```python
from build123d import *

# Parameters (mm, degrees)
PAD002_DEPTH              = 7.5
BODY002_PLACEMENT_ANGLE   = 90
CYLINDER015_R             = 4.5
CYLINDER015_DEPTH         = 9.5
COMPOUND_PLACEMENT_ANGLE  = 30
CYLINDER014_R             = 4.5
CYLINDER014_DEPTH         = 9.5
PAD001_DEPTH              = 4
BODY001_PLACEMENT_ANGLE   = 90
PAD_DEPTH                 = 7.5
BODY_PLACEMENT_ANGLE      = 90
CYLINDER016_R             = 2.25
CYLINDER016_DEPTH         = 9.5
BOX002_W                  = 58.914519
BOX002_H                  = 9.5
BOX002_DEPTH              = 15
BOX_W                     = 22
BOX_H                     = 9.5
BOX_DEPTH                 = 80.829038
CYLINDER013_R             = 11
CYLINDER013_DEPTH         = 9.5
CYLINDER012_R             = 11
CYLINDER012_DEPTH         = 9.5
FUSION005_PLACEMENT_ANGLE = 30
BOX001_W                  = 22
BOX001_H                  = 9.5
BOX001_DEPTH              = 50
FILLET_R                  = 2
FILLET001_R               = 2
FILLET002_R               = 2


with BuildPart() as m8press001:
    # Sketch002 → Pad002 (new body)
    with BuildSketch(Plane.XY):
        Polygon((7.5, 0), (3.75, 6.495191), (-3.75, 6.495191), (-7.5, 0), (-3.75, -6.495191), (3.75, -6.495191), align=None)
    extrude(amount=PAD002_DEPTH)


with BuildPart() as m8press001_1:
    # Body002 placement: moved
    add(m8press001.part.moved(Location((40.414519, -2, 70))).rotate(Axis((40.414519, -2, 70), (1, 0, 0)), BODY002_PLACEMENT_ANGLE))


with BuildPart() as compound:
    # Cylinder015 → Cylinder015 (new body)
    with BuildSketch(Plane(origin=(0, 0, 81), x_dir=(1, 0, 0), z_dir=(0, -1, 0))):
        Circle(CYLINDER015_R)
    extrude(amount=CYLINDER015_DEPTH)


with BuildPart() as compound_1:
    # Compound placement: moved
    add(compound.part.rotate(Axis((0, 0, 0), (0, 1, 0)), COMPOUND_PLACEMENT_ANGLE))


with BuildPart() as cylinder014:
    # Cylinder014 → Cylinder014 (new body)
    with BuildSketch(Plane.XZ):
        Circle(CYLINDER014_R)
    extrude(amount=CYLINDER014_DEPTH)


with BuildPart() as m4press:
    # Sketch001 → Pad001 (new body)
    with BuildSketch(Plane.XY):
        Polygon((4, 0), (2, 3.464102), (-2, 3.464102), (-4, 0), (-2, -3.464102), (2, -3.464102), align=None)
    extrude(amount=PAD001_DEPTH)


with BuildPart() as m4press_1:
    # Body001 placement: moved
    add(m4press.part.moved(Location((0, -5.5, 112.5))).rotate(Axis((0, -5.5, 112.5), (1, 0, 0)), BODY001_PLACEMENT_ANGLE))


with BuildPart() as m8press:
    # Sketch → Pad (new body)
    with BuildSketch(Plane.XY):
        Polygon((7.5, 0), (3.75, 6.495191), (-3.75, 6.495191), (-7.5, 0), (-3.75, -6.495191), (3.75, -6.495191), align=None)
    extrude(amount=PAD_DEPTH)


with BuildPart() as m8press_1:
    # Body placement: moved
    add(m8press.part.rotate(Axis((0, 0, 0), (1, 0, 0)), BODY_PLACEMENT_ANGLE))


with BuildPart() as fusion006:
    # Cylinder016 → Cylinder016 (new body)
    with BuildSketch(Plane(origin=(0, 0, 112.5), x_dir=(1, 0, 0), z_dir=(0, -1, 0))):
        Circle(CYLINDER016_R)
    extrude(amount=CYLINDER016_DEPTH)

    # Fusion006: union M8Press001, Compound, Cylinder014, M4Press, M8Press
    add(m8press001_1.part)
    add(compound_1.part)
    add(cylinder014.part)
    add(m4press_1.part)
    add(m8press_1.part)


with BuildPart() as cube002:
    # Box002 → Box002 (new body)
    with BuildSketch(Plane(origin=(-7.5, -9.5, 105), x_dir=(1, 0, 0), z_dir=(0, 0, 1))):
        with Locations((29.457259, 4.75)):
            Rectangle(BOX002_W, BOX002_H)
    extrude(amount=BOX002_DEPTH)


with BuildPart() as cube:
    # Box → Box (new body)
    with BuildSketch(Plane(origin=(-11, -9.5, 0), x_dir=(1, 0, 0), z_dir=(0, 0, 1))):
        with Locations((11, 4.75)):
            Rectangle(BOX_W, BOX_H)
    extrude(amount=BOX_DEPTH)


with BuildPart() as cylinder013:
    # Cylinder013 → Cylinder013 (new body)
    with BuildSketch(Plane(origin=(0, 0, 81), x_dir=(1, 0, 0), z_dir=(0, -1, 0))):
        Circle(CYLINDER013_R)
    extrude(amount=CYLINDER013_DEPTH)


with BuildPart() as fusion005:
    # Cylinder012 → Cylinder012 (new body)
    with BuildSketch(Plane.XZ):
        Circle(CYLINDER012_R)
    extrude(amount=CYLINDER012_DEPTH)

    # Fusion005: union Cube, Cylinder013
    add(cube.part)
    add(cylinder013.part)


with BuildPart() as fusion005_1:
    # Fusion005 placement: moved
    add(fusion005.part.rotate(Axis((0, 0, 0), (0, 1, 0)), FUSION005_PLACEMENT_ANGLE))


with BuildPart() as fillet002:
    # Box001 → Box001 (new body)
    with BuildSketch(Plane(origin=(29.414519, -9.5, 70), x_dir=(1, 0, 0), z_dir=(0, 0, 1))):
        with Locations((11, 4.75)):
            Rectangle(BOX001_W, BOX001_H)
    extrude(amount=BOX001_DEPTH)

    # Fusion007: union Cube002, Fusion005
    add(cube002.part)
    add(fusion005_1.part)

    # Cut005: cut Fusion006
    add(fusion006.part, mode=Mode.SUBTRACT)

    # Fillet
    fillet_edges = [fillet002.edges().sort_by_distance(p)[0] for p in [
        (51.414519, -4.75, 120),
        (-7.5, -4.75, 105),
        (-7.5, -4.75, 120),
    ]]
    fillet(fillet_edges, radius=FILLET_R)

    # Fillet001
    fillet001_edges = [fillet002.edges().sort_by_distance(p)[0] for p in [
        (29.414519, -4.75, 105),
    ]]
    fillet(fillet001_edges, radius=FILLET001_R)

    # Fillet002
    fillet002_edges = [fillet002.edges().sort_by_distance(p)[0] for p in [
        (29.414519, -4.75, 72.947441),
    ]]
    fillet(fillet002_edges, radius=FILLET002_R)


solid = fillet002.part
```
Build history of the part. All positions in model axes, mm. A direction names the side the tool comes from. Coordinates: 2 decimals unless noted, no trailing zeros. Order: outer loops, then holes, each group sorted by start corner. A loop starts at its lowest first (then second) coordinate and runs counter-clockwise, first axis right, second up. Notation, with made-up numbers: (30.5, -6) -> (44.5, -6) arc R35 ccw to (44.5, 28) -> close; hole circle Ø8 at (43.5, 47). An arc over 180 degrees is marked (long way). Answer in a Markdown table with one row per item. Add a question column.
Q1. Wall check: line 1 along Z through (x, y) = (21, -2.25); line 2 along X through (y, z) = (-3.25, 112); line 3 along Z through (x, y) = (40.5, -7). Give the ranges that are in metal, low to high. Write a range as [from, to].
Q2. Mould opens along Z. For faces 5 (the face through (22, -5, 120)), 6 (the face through (29.45, -4.82, 29.01)), 7 (the face through (2, -5.5, 111)) say: +Z half, -Z half, draft (parallel to the pull), parting line (faces both ways), or undercut.
Q3. Band-saw the part on D-D, the plane x = 42.5. List the corners of the cut face in (y, z), then the cut area to 3 significant figures.
Q4. Band-saw the part on C-C, the plane z = 94. List the corners of the cut face in (x, y).
Q5. Drop flat-ended pins along their axis: pin 1 (5.5 mm diameter, centred on x = -1.5, z = 111.5, fed in from -Y); pin 2 (5 mm diameter, centred on x = 32, y = -3.5, fed in from -Z); pin 3 (5 mm diameter, centred on y = -8.5, z = 31, fed in from -X); pin 4 (3 mm diameter, centred on y = -2, z = 37.5, fed in from -X). Give the stop position or say it passes through.
Q6. Band-saw the part on A-A, the plane x = 0. List the corners of the cut face in (y, z), then the cut area to 3 significant figures.
Q7. Band-saw the part on B-B, the plane x = 20. List the corners of the cut face in (y, z), then the cut area to 4 significant figures.
Q8. Which spindle directions (+Z, -Z, +X, -X, +Y, -Y) get a long thin tool onto all of the face, cutting with end or side? Do faces 1 (the face through (-5.651, -3.698, -3.202)), 2 (the face through (40, -6, 63.505)), 3 (the face through (9.54, -4.82, 38.52)), 4 (the face through (51.254, -4.684, 67.835)). Say none if no direction does.
Answers follow:
| question | item | result |
|---|---|---|
| 1 | line 1 | [14.37, 58.37], [105, 120] |
| 1 | line 2 | [-7.5, -2.19], [2.19, 51.41] |
| 1 | line 3 | [48.15, 63.5], [76.5, 120] |
| 2 | face 5 | +Z half |
| 2 | face 6 | -Z half |
| 2 | face 7 | undercut |
| 3 | outline | (-9.5, 51.61) -> (0, 51.61) -> (0, 66.12) -> (-2, 66.12) -> (-2, 63.5) -> (-9.5, 63.5) -> close; (-9.5, 76.5) -> (-2, 76.5) -> (-2, 74.18) -> (0, 74.18) -> (0, 120) -> (-9.5, 120) -> close |
| 3 | area | 536 mm^2 |
| 4 | outline | (29.41, -9.5) -> (51.41, -9.5) -> (51.41, 0) -> (29.41, 0) -> close |
| 5 | pin 1 | y = -9.5 |
| 5 | pin 2 | z = 29.1 |
| 5 | pin 3 | x = 3.75 |
| 5 | pin 4 | x = 8.08 |
| 6 | outline | (-9.5, -11) -> (0, -11) -> (0, -6.5) -> (-7.5, -6.5) -> (-7.5, -4.5) -> (-9.5, -4.5) -> close; (-9.5, 4.5) -> (-7.5, 4.5) -> (-7.5, 6.5) -> (0, 6.5) -> (0, 22) -> (-9.5, 22) -> close; (-9.5, 105) -> (0, 105) -> (0, 110.25) -> (-5.5, 110.25) -> (-5.5, 109.04) -> (-9.5, 109.04) -> close; (-9.5, 115.96) -> (-5.5, 115.96) -> (-5.5, 114.75) -> (0, 114.75) -> (0, 120) -> (-9.5, 120) -> close |
| 6 | area | 288 mm^2 |
| 7 | outline | (-9.5, 12.64) -> (0, 12.64) -> (0, 56.64) -> (-9.5, 56.64) -> close; (-9.5, 105) -> (0, 105) -> (0, 120) -> (-9.5, 120) -> close |
| 7 | area | 560.5 mm^2 |
| 8 | face 1 | +Y |
| 8 | face 2 | -Y |
| 8 | face 3 | -X, +Y, -Y |
| 8 | face 4 | +X, +Y, -Y |
